CAD build for the part. Positions are in the model's coordinates, mm. A direction names the side the tool comes from. Give positions to 0.01 mm unless a question says otherwise; leave off trailing zeros. Order: outer loops, then holes, each group sorted by start corner. A loop starts at its lowest first (then second) coordinate and runs counter-clockwise, first axis right, second up.
Item 1: Band-saw the part on D-D on y = -9.5. Give the cut face in (x, z).
Item 2: Flat gauge pin, fed straight in: P1, Ø5, axis at x = -13.5, z = 11.5, coming from the +Y side. Where does the tip first touch, or does it go through?
Item 3: Band-saw the part on C-C on y = -40. Give the cut face in (x, z), plus the area to 4 significant figures.
Item 4: Band-saw the part on B-B on x = -16. Give the cut face in (y, z).
Item 5: Wall check: L1, parallel to Z at x = 5, y = -7; L2, parallel to X at y = -24, z = -2.5; L3, parallel to Z at x = 28.7, y = -40. Give the ranges that are in metal, low to high.
Item 6: Band-saw the part on A-A on z = -5.5. Give the cut face in (x, y).
Item 7: Two-plate mould, pull along Y, no slides. Class faces 1 (the cylindrical face through (28.732, -24.003, -4.869)), 2 (the flat face through (0, -50, 0)), 3 (the flat face through (0, -25, -17.5)): released by +Y, released by -Y, zero draft, split by the parting line, or undercut.
Item 8: Which spindle directions (+Z, -Z, +X, -X, +Y, -Y) get a long thin tool onto all of the face, cutting with end or side? Do faces 4 (the flat face through (0, -23, -15)), 5 (the cylindrical face through (28.732, -22.003, 6.131)), 6 (the flat face through (30, -25, 0)). Say none if no direction does.
```python
from build123d import *

# Parameters (mm, degrees)
F0_W     = 60
F0_H     = 35
F1_DEPTH = 50
F2_T     = -2.5
F4_D     = 4.2
F4_DEPTH = 14.4
F4_TIP   = 1.2618073


with BuildPart() as f1:
    # F0 (on Front) → F1 (new body)
    with BuildSketch(Plane.XZ):
        Rectangle(F0_W, F0_H)
    extrude(amount=F1_DEPTH)

    # F2
    f2_openings = [f1.faces().sort_by_distance(p)[0] for p in [
        (0, 0, 0),
    ]]
    offset(amount=F2_T, openings=f2_openings)

    # F4
    with Locations(Plane.YZ.offset(30)):
        with Locations((-40, -0.5), (-20, 5.5), (-22, -5.5)):
            Hole(F4_D / 2, depth=F4_DEPTH)
            with Locations((0, 0, -(F4_DEPTH + F4_TIP / 2))):  # 118° drill point
                Cone(0, F4_D / 2, F4_TIP, mode=Mode.SUBTRACT)


solid = f1.part
```
The answers:
1. outline: (-30, -17.5) - (30, -17.5) - (30, 17.5) - (-30, 17.5) - close; hole (-27.5, -15) - (27.5, -15) - (27.5, 15) - (-27.5, 15) - close
2. P1: stops at y = -47.5
3. outline: (-30, -17.5) - (30, -17.5) - (30, -2.6) - (27.5, -2.6) - (27.5, -15) - (-27.5, -15) - (-27.5, 15) - (27.5, 15) - (27.5, 1.6) - (30, 1.6) - (30, 17.5) - (-30, 17.5) - close
3. area: 439.5 mm2
4. outline: (-50, -17.5) - (0, -17.5) - (0, -15) - (-47.5, -15) - (-47.5, 15) - (0, 15) - (0, 17.5) - (-50, 17.5) - close
5. L1: z = -17.5 to -15, 15 to 17.5
5. L2: x = -30 to -27.5, 27.5 to 30
5. L3: z = -17.5 to -2.6, 1.6 to 17.5
6. outline: (-30, -50) - (30, -50) - (30, -24.1) - (27.5, -24.1) - (27.5, -47.5) - (-27.5, -47.5) - (-27.5, 0) - (-30, 0) - close; (27.5, -19.9) - (30, -19.9) - (30, 0) - (27.5, 0) - close
7. face 1: undercut
7. face 2: released by -Y
7. face 3: zero draft
8. face 4: +Y
8. face 5: +X
8. face 6: +Z, -Z, +X, +Y, -Y
